from build123d import *

# Parameters (mm, degrees)
BOSS_EXTRUDE1_DEPTH     = 15
CUT_EXTRUDE1_DEPTH      = 13.5
SKETCH3_W               = 13.5
SKETCH3_H               = 27
CUT_EXTRUDE2_DEPTH      = 15
SALIENTE_EXTRUIR1_DEPTH = 2


with BuildPart() as part:
    # Sketch1 → Boss-Extrude1 (new body)
    with BuildSketch(Plane(origin=(0, 0, 0), x_dir=(1, 0, 0), z_dir=(0, 1, 0))):
        with BuildLine():
            Line((-21.75, -50), (21.75, -50))
            ThreePointArc((21.75, -50), (24.224873734, -48.974873734), (25.25, -46.5))
            Line((25.25, -46.5), (25.25, 46.5))
            ThreePointArc((25.25, 46.5), (24.224873734, 48.974873734), (21.75, 50))
            Line((21.75, 50), (-21.75, 50))
            ThreePointArc((-21.75, 50), (-24.224873734, 48.974873734), (-25.25, 46.5))
            Line((-25.25, 46.5), (-25.25, -46.5))
            ThreePointArc((-25.25, -46.5), (-24.224873734, -48.974873734), (-21.75, -50))
        make_face()
    extrude(amount=BOSS_EXTRUDE1_DEPTH)

    # Sketch2 → Cut-Extrude1 (cut)
    with BuildSketch(Plane.XZ):
        with BuildLine():
            Line((-19.75, -48), (19.75, -48))
            ThreePointArc((19.75, -48), (22.224873734, -46.974873734), (23.25, -44.5))
            Line((23.25, -44.5), (23.25, 44.5))
            ThreePointArc((23.25, 44.5), (22.224873734, 46.974873734), (19.75, 48))
            Line((19.75, 48), (-19.75, 48))
            ThreePointArc((-19.75, 48), (-22.224873734, 46.974873734), (-23.25, 44.5))
            Line((-23.25, 44.5), (-23.25, -44.5))
            ThreePointArc((-23.25, -44.5), (-22.224873734, -46.974873734), (-19.75, -48))
        make_face()
    extrude(amount=-CUT_EXTRUDE1_DEPTH, mode=Mode.SUBTRACT)

    # Sketch3 → Cut-Extrude2 (cut)
    with BuildSketch(Plane.XY.offset(50)):
        Rectangle(SKETCH3_W, SKETCH3_H)
    extrude(amount=-CUT_EXTRUDE2_DEPTH, mode=Mode.SUBTRACT)

    # Croquis3 → Saliente-Extruir1 (add)
    with BuildSketch(Plane.XZ):
        with BuildLine():
            Line((7.25, 48.5), (19.75, 48.5))
            ThreePointArc((19.75, 48.5), (22.578427125, 47.328427125), (23.75, 44.5))
            Line((23.75, 44.5), (23.75, -44.5))
            ThreePointArc((23.75, -44.5), (22.578427125, -47.328427125), (19.75, -48.5))
            Line((19.75, -48.5), (-19.75, -48.5))
            ThreePointArc((-19.75, -48.5), (-22.578427125, -47.328427125), (-23.75, -44.5))
            Line((-23.75, -44.5), (-23.75, 44.5))
            ThreePointArc((-23.75, 44.5), (-22.578427125, 47.328427125), (-19.75, 48.5))
            Line((-19.75, 48.5), (-7.25, 48.5))
            Line((-7.25, 48.5), (-7.25, 49.5))
            Line((-7.25, 49.5), (-21.75, 49.5))
            ThreePointArc((-21.75, 49.5), (-23.871320344, 48.621320344), (-24.75, 46.5))
            Line((-24.75, 46.5), (-24.75, -46.5))
            ThreePointArc((-24.75, -46.5), (-23.871320344, -48.621320344), (-21.75, -49.5))
            Line((-21.75, -49.5), (21.75, -49.5))
            ThreePointArc((21.75, -49.5), (23.871320344, -48.621320344), (24.75, -46.5))
            Line((24.75, -46.5), (24.75, 46.5))
            ThreePointArc((24.75, 46.5), (23.871320344, 48.621320344), (21.75, 49.5))
            Line((21.75, 49.5), (7.25, 49.5))
            Line((7.25, 49.5), (7.25, 48.5))
        make_face()
    extrude(amount=SALIENTE_EXTRUIR1_DEPTH)


solid = part.part
Check sheet for the modelled part. Datum: model origin and axes. Units: mm. A direction names the side the tool comes from. Round coordinates to 2 decimals unless told otherwise and drop trailing zeros. Order: outer loops, then holes, each group sorted by start corner. A loop starts at its lowest first (then second) coordinate and runs counter-clockwise, first axis right, second up.
Q1. Set-up check for faces 1 (the face through (6.75, 7, 49)), 2 (the face through (23.25, 7, -1)), 3 (the face through (23.89, -0.99, 48.6)), 4 (the face through (23.85, -0.99, -48.64)): record each of +Z, -Z, +X, -X, +Y, -Y from which the full face is reachable in a straight line by a thin tool's end or side.
Filled sheet:
face 1: +Z, -Y
face 2: -Y
face 3: +Z, +X, -Y
face 4: -Z, +X, -Y
Q2. Cross-section at C-C, the plane z = -24.5. Enter the section's corners in (x, y), plus the area to 3 significant figures.
Filled sheet:
outline: (-25.25, 0) - (-24.75, 0) - (-24.75, -2) - (-23.75, -2) - (-23.75, 0) - (-23.25, 0) - (-23.25, 13.5) - (23.25, 13.5) - (23.25, 0) - (23.75, 0) - (23.75, -2) - (24.75, -2) - (24.75, 0) - (25.25, 0) - (25.25, 15) - (-25.25, 15) - close
area: 134 mm2
Q3. Depth check by flat-ended pin: P1, Ø4, axis at x = -2.5, y = 9.5, coming from the +Z side; P2, Ø0.8, axis at y = -1, z = 49, coming from the +X side; P3, Ø6, axis at x = -1, z = 34, coming from the -Y side. Enter the tip coordinate at first touch or a pass-through.
Filled sheet:
P1: stops at z = -48
P2: stops at x = 23.89
P3: stops at y = 13.5
Q4. Scan lines: L1, parallel to X at y = 10.25, z = 12; L2, parallel to Z at x = -20, y = 9.25; L3, parallel to X at y = -1, z = 37.5. Record each from-to range of solid material in increasing order.
Filled sheet:
L1: x = -25.25 to -23.25, 23.25 to 25.25
L2: z = -50 to -47.99, 47.99 to 50
L3: x = -24.75 to -23.75, 23.75 to 24.75
Q5. Cross-section at B-B, the plane x = -9.5. Enter the section's corners in (y, z), plus the area to 3 significant figures.
Filled sheet:
outline: (-2, -49.5) - (0, -49.5) - (0, -50) - (15, -50) - (15, 50) - (0, 50) - (0, 49.5) - (-2, 49.5) - (-2, 48.5) - (0, 48.5) - (0, 48) - (13.5, 48) - (13.5, -48) - (0, -48) - (0, -48.5) - (-2, -48.5) - close
area: 208 mm2
Q6. Cross-section at A-A, the plane y = 10.25. Enter the section's corners in (x, z).
Filled sheet:
outline: (-25.25, -46.5) arc R3.5 ccw to (-21.75, -50) - (21.75, -50) arc R3.5 ccw to (25.25, -46.5) - (25.25, 46.5) arc R3.5 ccw to (21.75, 50) - (6.75, 50) - (6.75, 48) - (19.75, 48) arc R3.5 cw to (23.25, 44.5) - (23.25, -44.5) arc R3.5 cw to (19.75, -48) - (-19.75, -48) arc R3.5 cw to (-23.25, -44.5) - (-23.25, 44.5) arc R3.5 cw to (-19.75, 48) - (-6.75, 48) - (-6.75, 50) - (-21.75, 50) arc R3.5 ccw to (-25.25, 46.5) - close
Q7. Cross-section at D-D, the plane x = 5. Enter the section's corners in (y, z).
Filled sheet:
outline: (-2, -49.5) - (0, -49.5) - (0, -50) - (15, -50) - (15, 50) - (13.5, 50) - (13.5, -48) - (0, -48) - (0, -48.5) - (-2, -48.5) - close
